The listing builds one solid part. Answer for the finished solid, in the listing's coordinates (mm). Face numbers are marked on the shaded views. A direction names the side the tool comes from. Coordinates: 2 decimals unless noted, no trailing zeros. Order: outer loops, then holes, each group sorted by start corner. A loop starts at its lowest first (then second) coordinate and runs counter-clockwise, first axis right, second up. Notation, with made-up numbers: (72.5, 30.5) -> (129.5, 30.5) arc R17 cw to (129.5, 55.5) -> close; hole circle Ø3 at (-32, 87.5). An arc over 180 degrees is marked (long way). Answer in a Markdown table with one row per item.
Autodesk Inventor part; units mm, degrees
ref_plane "YZ Plane" through (0, 0, 0) normal (1, 0, 0) x (0, 1, 0)
ref_plane "XZ Plane" through (0, 0, 0) normal (0, 1, 0) x (-1, 0, 0)
ref_plane "XY Plane" through (0, 0, 0) normal (0, 0, 1) x (1, 0, 0)
sketch "Sketch1" plane through (0, 0, 0) normal (0, 1, 0) x (-1, 0, 0)
  line L0 (-0.2883, 0) -> (44.7117, 0)
  line L1 (44.7117, 0) -> (44.7117, 30)
  line L2 (44.7117, 30) -> (-0.2883, 30)
  line L3 (-0.2883, 30) -> (-0.2883, 0)
  point P0 (0, 0)
  dimension "d0" = 45
  dimension "d1" = 30
extrude "Extrusion1" add sketch "Sketch1" along normal blind 30
sketch "Sketch2" plane through (-44.7117, 0, 0) normal (-1, 0, 0) x (0, 0, 1)
  line L0 (19.294, 8.1716) -> (10.706, 21.8284) construction
  line L1 (10.706, 8.1716) -> (19.294, 21.8284) construction
  line L2 (17.5, 10) -> (12.5, 10)
  line L3 (12.5, 10) -> (12.5, 20)
  line L4 (12.5, 20) -> (17.5, 20)
  line L5 (17.5, 20) -> (17.5, 10)
  line L6 (17.5, 10) -> (12.5, 20) construction
  line L7 (12.5, 10) -> (17.5, 20) construction
  line L8 (12.5, 10) -> (7.5, 10)
  line L9 (7.5, 10) -> (7.5, 20)
  line L10 (7.5, 20) -> (12.5, 20)
  line L11 (12.5, 20) -> (12.5, 10)
  line L12 (17.5, 10) -> (22.5, 10)
  line L13 (22.5, 10) -> (22.5, 20)
  line L14 (22.5, 20) -> (17.5, 20)
  line L15 (17.5, 20) -> (17.5, 10)
  point P0 (0, 0)
  point P1 (15, 15)
  dimension "d4" = 5
  dimension "d5" = 10
  dimension "d6" = 5
  dimension "d7" = 5
extrude "Extrusion2" add sketch "Sketch2" along normal blind 9 contours L5 L14 L13 L12 | L8 L9 L10 L3
sketch "Sketch3" plane through (-44.7117, 10, 7.5) normal (0, 0, -1) x (-1, 0, 0)
  line L0 (0, -10) -> (0, 20)
  line L1 (0, 5) -> (5, 5)
  circle A0 centre (5, 5) radius 2.5
  point P0 (-44.7117, -10)
  dimension "d10" = 5
  dimension "d11" = 5
extrude "Extrusion3" cut sketch "Sketch3" against normal through all
sketch "Sketch4" plane through (0.2883, 0, 30) normal (1, 0, 0) x (0, 0, -1)
  line L0 (12.5, 10) -> (12.5, 20)
  line L1 (17.5, 10) -> (22.5, 10)
  line L2 (12.5, 20) -> (17.5, 20)
  line L3 (17.5, 20) -> (17.5, 10)
  line L4 (17.5, 10) -> (12.5, 10)
  line L5 (12.5, 10) -> (12.5, 20)
  line L6 (17.5, 20) -> (22.5, 20)
  line L7 (17.5, 10) -> (22.5, 10)
  line L8 (22.5, 10) -> (22.5, 20)
  line L9 (22.5, 20) -> (17.5, 20)
  line L10 (17.5, 20) -> (17.5, 10)
  line L11 (7.5, 10) -> (12.5, 10)
  line L12 (12.5, 20) -> (7.5, 20)
  line L13 (7.5, 20) -> (7.5, 10)
  line L14 (7.5, 10) -> (12.5, 10)
  line L15 (12.5, 10) -> (12.5, 20)
  point P0 (30, 0)
extrude "Extrusion4" add sketch "Sketch4" along normal blind 10 contours L11 L13 L12 L0 | L3 L6 L8 L1
sketch "Sketch5" plane through (0.2883, 10, 12.5) normal (0, 0, 1) x (-1, 0, 0)
  line L0 (0, 10) -> (0, -20)
  line L1 (0, -5) -> (-5, -5)
  circle A0 centre (-5, -5) radius 2.5
  point P0 (0.2883, 10)
  dimension "d16" = 5
  dimension "d17" = 5
extrude "Extrusion5" cut sketch "Sketch5" against normal through all
sketch "Sketch6" plane through (-44.7117, 0, 30) normal (0, 0, 1) x (1, 0, 0)
  circle A0 centre (22.5, 15) radius 2.5
  line L0 (0, 0) -> (0, 30)
  point P0 (44.7117, 0)
  point P1 (0, 15)
  dimension "d20" = 5
  dimension "d23" = 22.5
extrude "Extrusion6" cut sketch "Sketch6" against normal blind 5
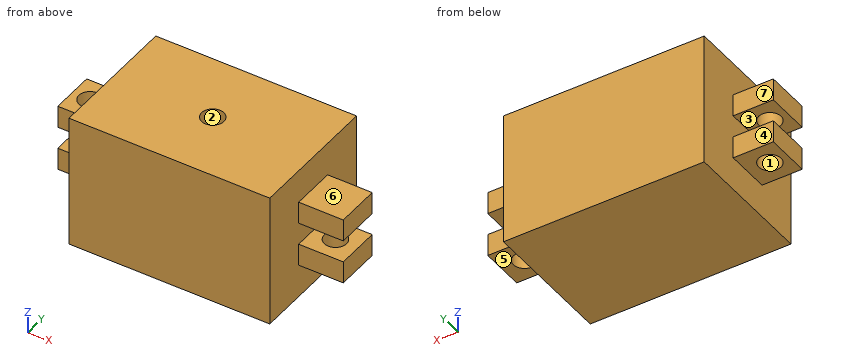
(1) For a pull along Y with two mould halves and no side action, classify the marked faces 1, 2, 3 and 4 as released by +Y, released by -Y, zero draft, split by the parting line, or undercut.
Check values:
| item | result |
|---|---|
| face 1 | undercut |
| face 2 | undercut |
| face 3 | zero draft |
| face 4 | released by +Y |
(2) Flat-ended cylindrical pins translate along their axes: pin 1 (10 mm diameter, centred on x = -50.5, y = 12.5, fed in from -Z); pin 2 (1.5 mm diameter, centred on x = 5, z = 21, fed in from +Y); pin 3 (5.5 mm diameter, centred on x = 5, z = 9.5, fed in from -Y). Find the tip coordinate at first contact, or state that the pin passes through.
Check values:
| item | result |
|---|---|
| pin 1 | z = 7.5 |
| pin 2 | y = 20 |
| pin 3 | y = 10 |
(3) Which of the six approach directions +Z, -Z, +X, -X, +Y, -Y give full straight-line access (tool end or side, diameter ignored) to the marked faces 5, 6 and 7?
Check values:
| item | result |
|---|---|
| face 5 | -Z, +X, +Y, -Y |
| face 6 | +Z, +X, +Y, -Y |
| face 7 | +Z, -Z, -X, +Y |
(4) A cutting plane is placed at A-A, the plane z = 21. Determine the outline of the cut face in (x, y).
Check values:
| item | result |
|---|---|
| outline | (-53.71, 10) -> (-44.71, 10) -> (-44.71, 0) -> (0.29, 0) -> (0.29, 10) -> (10.29, 10) -> (10.29, 20) -> (0.29, 20) -> (0.29, 30) -> (-44.71, 30) -> (-44.71, 20) -> (-53.71, 20) -> close; hole circle Ø5 at (-49.71, 15) |
(5) A cutting plane is placed at C-C, the plane y = 4. Determine the outline of the cut face in (x, z).
Check values:
| item | result |
|---|---|
| outline | (-44.71, 0) -> (0.29, 0) -> (0.29, 30) -> (-44.71, 30) -> close |
(6) A cutting plane is placed at B-B, the plane y = 15. Count the separate pieces of the cut face and the enclosed holes in it, then the cut area to 3 significant figures.
Check values:
| item | result |
|---|---|
| separate pieces | 4 |
| enclosed holes | 0 |
| area | 1,440 mm² |
(7) Find the intervals of material crossed by line 1 along X through (y, z) = (15, 10.5); line 2 along Z through (x, y) = (-49.5, 19.25); line 3 along X through (y, z) = (15, 19.6), in increasing order. Write a range as from..to.
Check values:
| item | result |
|---|---|
| line 1 | -53.71..-52.21, -47.21..2.79, 7.79..10.29 |
| line 2 | 7.5..12.5, 17.5..22.5 |
| line 3 | -53.71..-52.21, -47.21..10.29 |
